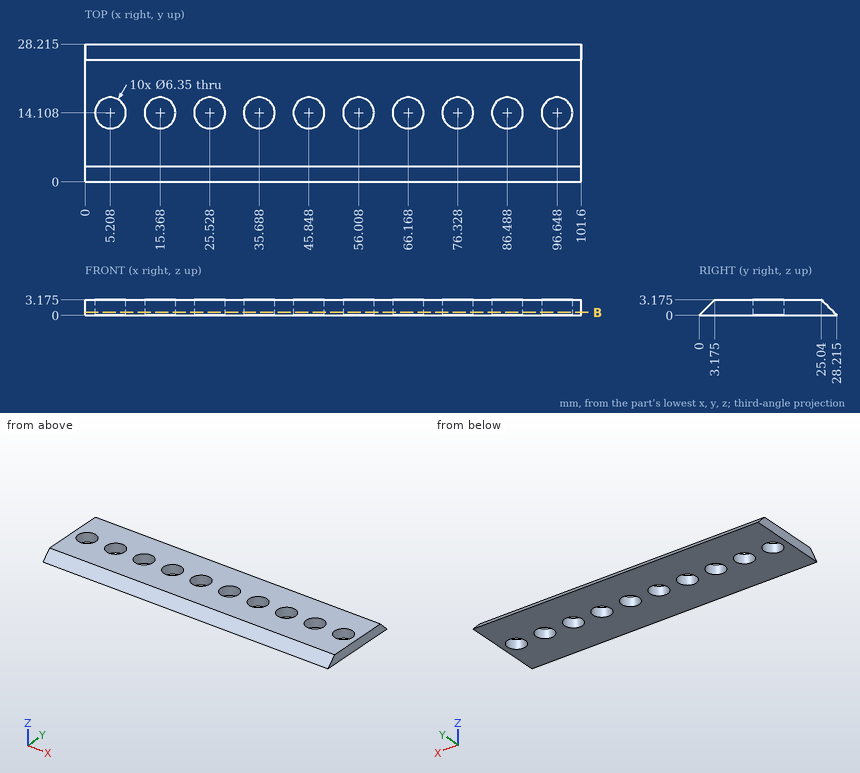
Input: dimensioned drawing with shaded views. Units: mm. Origin: part minimum x, y, z. Coordinates: 2 decimals unless noted, no trailing zeros. One line per item, written item: value. Start each with the question number.
Q1. Section query B-B, the plane z = 0.6. Give the number of separate pieces and of enclosed holes in the cut face, and give its area (3 significant figures).
Q2. Line query: line 1 along Y through (x, z) = (78.5, 0.3) (1 decimal); line 2 along Y through (x, z) = (56, 1.3) (1 decimal); line 3 along Z through (x, y) = (58, 2.25). Output: solid intervals per line, ascending.
Q3. Contact query for flat-ended pins moving along their axis: P1, Ø1, axis at x = 43, z = 1, coming from the +Y side (1 decimal); P2, Ø5.5, axis at x = 66.17, y = 14.11, coming from the -Z side; P3, Ø10, axis at x = 76.33, y = 14.11, coming from the +Z side (3 decimals); P4, Ø1, axis at x = 54.5, z = 2.5, coming from the -Y side. Output: stop coordinate, or through.
Results:
1. separate pieces: 1
1. enclosed holes: 10
1. area: 2,430 mm^2
2. line 1: 0.3 to 11.8, 16.4 to 27.9
2. line 2: 1.3 to 10.9, 17.3 to 26.9
2. line 3: 0 to 2.25
3. P1: y = 27.7
3. P2: through
3. P3: z = 3.175
3. P4: y = 2
